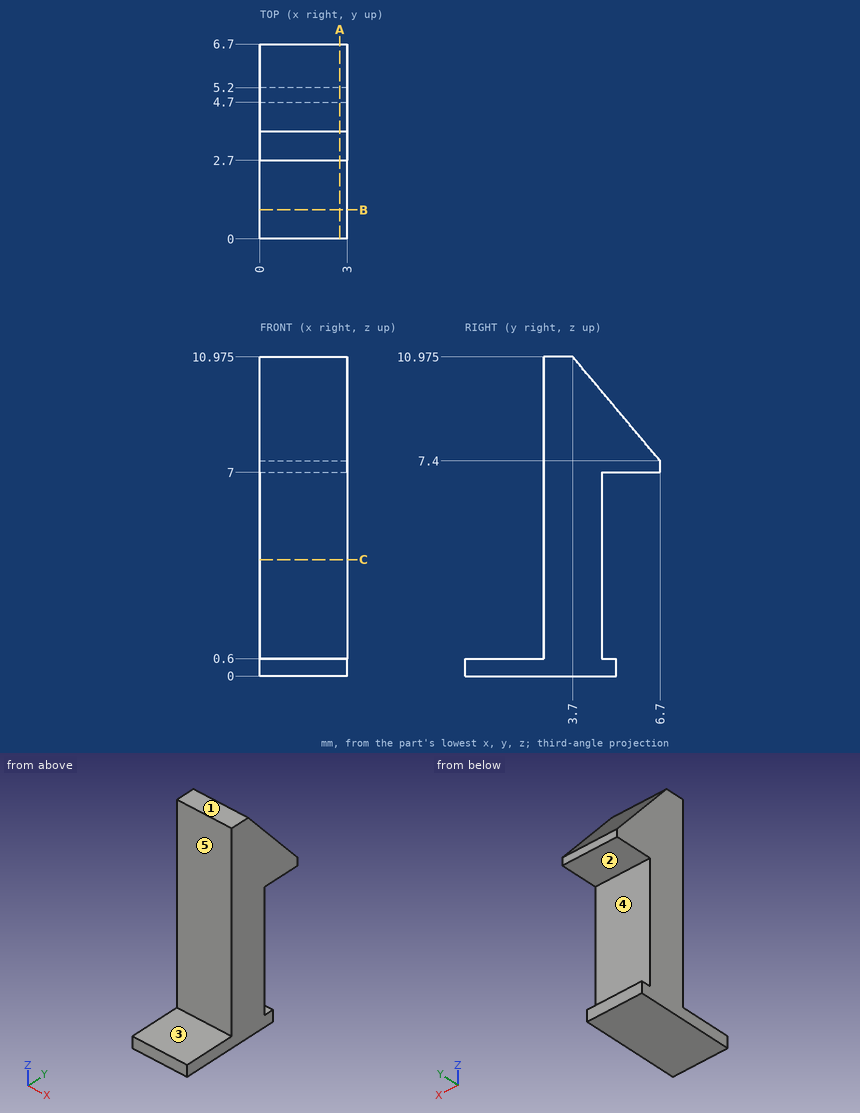
Geometry check sheet. Reference: drawing and pictorial views, mm from the part's lowest x, y, z. A direction names the side the tool comes from. Coordinates: 2 decimals unless noted, no trailing zeros. Loops run counter-clockwise (first coordinate to the right, second up) from the corner with the lowest first, then second, coordinate; pieces in that order, holes last. Notation, with made-up numbers: (-23, 56) -> (10, 56) arc R23 ccw to (10, 67) -> close; hole circle Ø8 at (77.5, 24.25). An arc over 180 degrees is marked (long way). Put each result on its own line as item: value.
1) Cross-section at B-B on y = 1. Record the boundary of the cut face in (x, z), plus the area to 3 significant figures.
Result set:
outline: (0, 0) -> (3, 0) -> (3, 0.6) -> (0, 0.6) -> close
area: 1.80 mm^2
2) Cross-section at C-C on z = 4. Record the boundary of the cut face in (x, y).
Result set:
outline: (0, 2.7) -> (3, 2.7) -> (3, 4.7) -> (0, 4.7) -> close
3) Tool access check on the marked faces 1 and 2. Record the directions out of +Z, -Z, +X, -X, +Y, -Y that give a thin tool (end or side, any length) a straight path to the whole face; none if there is none.
Result set:
face 1: +Z, +X, -X, +Y, -Y
face 2: +X, -X, +Y
4) Release check for a two-part mould opening along Z. For the marked faces 3, 4 and 5 record: released by +Z, released by -Z, zero draft, split by the parting line, or undercut.
Result set:
face 3: released by +Z
face 4: undercut
face 5: zero draft
5) Gauge pin test, flat ends, axial feed: pin 1 Ø1.5 at (x, z) = (2, 8.5) entering from -Y; pin 2 Ø2 at (y, z) = (2, 5) entering from -X; pin 3 Ø0.5 at (x, z) = (2, 0.5) entering from +Y. Record the tip position at first contact, or that the pin passes through.
Result set:
pin 1: stops at y = 2.7
pin 2: stops at x = 0
pin 3: stops at y = 5.2
6) Cross-section at A-A on x = 2.75. Record the boundary of the cut face in (y, z) (1 decimal).
Result set:
outline: (0, 0) -> (5.2, 0) -> (5.2, 0.6) -> (4.7, 0.6) -> (4.7, 7) -> (6.7, 7) -> (6.7, 7.4) -> (3.7, 11) -> (2.7, 11) -> (2.7, 0.6) -> (0, 0.6) -> close
7) Thickness scan on line 1 (Y direction, x = 1, z = 5.5); line 2 (Z direction, x = 1, y = 1.25); line 3 (Y direction, x = 2.5, z = 7.25). Record the ranges inside material, lowest first.
Result set:
line 1: y = 2.7 to 4.7
line 2: z = 0 to 0.6
line 3: y = 2.7 to 6.7
